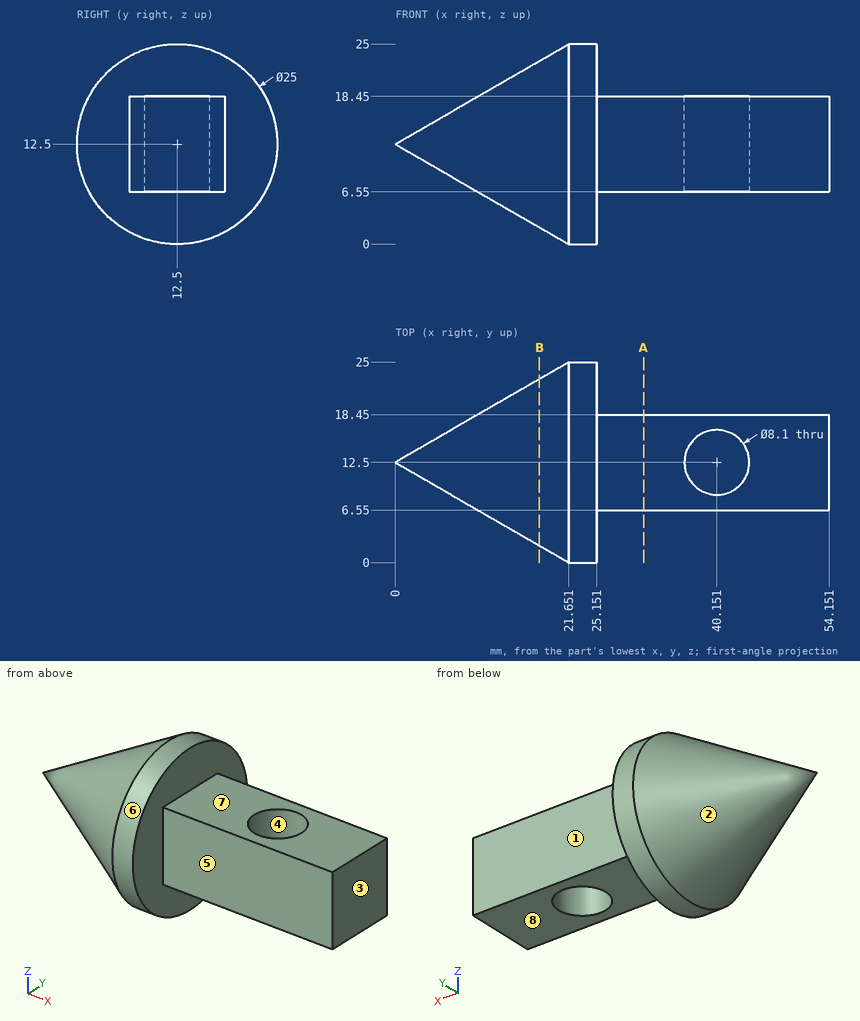
Part print with two shaded views. Sizes in mm from the minimum x, y, z corner. A direction names the side the tool comes from. Round coordinates to 2 decimals unless told otherwise and drop trailing zeros. Write each loop counter-clockwise with the first axis right and the second up, starting at its lowest first coordinate (ties: lowest second). Pieces come first, ordered by that corner, then holes. Notation, with made-up numbers: M -10.75,33 L 38.25,33 A22 cw 38.25,46 Z; hole C -24,-8 d4. An arc over 180 degrees is marked long. Put each result on its own line as item: value. Start each with the question number.
1) Saw through at B-B, the plane x = 18. Write the cut outline in (y, z) (1 decimal), and give its area (3 significant figures).
2) 3-axis set-ups, long thin cutter, end or side, ignore diameter. For the marked faces 5, 6, 7 and 8: which of +Z, -Z, +X, -X, +Y, -Y reach the whole face in a straight line?
3) Drill centre lines: probe 1 along Y at (x, z) = (40, 17); probe 2 along Y at (x, z) = (34, 7.75). Where is each one in solid material? Low to high. Write a range as [from, to].
4) Pull direction X, two halves, no side cores. Call the marked faces 1, 2, 3 and 4: pulls with the +X half, pulls with the -X half, needs draft (parallel to the pull), parting line crosses it, or undercut.
5) Pin check, flat tips, straight feed: pin 1 Ø5 at (x, y) = (32, 4.5) entering from -Z; pin 2 Ø4 at (x, z) = (10, 10.5) entering from +Y; pin 3 Ø4 at (x, z) = (18, 14) entering from -Y; pin 4 Ø10 at (y, z) = (13.5, 3) entering from +X. Stop position of each tip, or through.
6) Saw through at A-A, the plane x = 31. Write the cut outline in (y, z).
Resolved:
1. outline: C 12.5,12.5 d20.8
1. area: 339 mm²
2. face 5: +Z, -Z, +X, -Y
2. face 6: +X, -X
2. face 7: +Z, +X, +Y, -Y
2. face 8: -Z, +X, +Y, -Y
3. probe 1: [6.55, 8.45], [16.55, 18.45]
3. probe 2: [6.55, 18.45]
4. face 1: needs draft
4. face 2: pulls with the -X half
4. face 3: pulls with the +X half
4. face 4: undercut
5. pin 1: z = 6.55
5. pin 2: y = 19.23
5. pin 3: y = 1.03
5. pin 4: x = 54.15
6. outline: M 6.55,6.55 L 18.45,6.55 L 18.45,18.45 L 6.55,18.45 Z
